from build123d import *

# Parameters (mm, degrees)
F0_W     = 10
F0_H     = 41.6184230894
F0_H_2   = 20
F1_DEPTH = 150
F2_W     = 6.3547044992
F2_H     = 150
F2_W_2   = 6.8435370922
F2_H_2   = 86.8458472192
F3_DEPTH = 25


with BuildPart() as f1:
    # F0 (on Top) → F1 (new body)
    with BuildSketch(Plane.XY):
        with Locations((-14.8092108965, -1.3289477304)):
            Rectangle(F0_W, F0_H)
        with Locations((-14.8092108965, -32.1381592751)):
            Rectangle(F0_W, F0_H_2)
    extrude(amount=F1_DEPTH)

    # F2 (on face) → F3 (join)
    with BuildSketch(Plane.YZ.offset(-9.8092108965)):
        with Locations((10.3059485555, 75)):
            Rectangle(F2_W, F2_H)
        with Locations((-32.4661172926, 106.5770763904)):
            Rectangle(F2_W_2, F2_H_2)
    extrude(amount=F3_DEPTH)


solid = f1.part
Read the model definition and answer for the solid it produces. Units are mm, in the model's axes. A direction names the side the tool comes from. Coordinates: 2 decimals unless noted, no trailing zeros. Order: outer loops, then holes, each group sorted by start corner. A loop starts at its lowest first (then second) coordinate and runs counter-clockwise, first axis right, second up. Notation, with made-up numbers: M 44,10.25 L 92,10.25 A24 ccw 92,48.25 Z; hole C 51.5,18 d11. An arc over 180 degrees is marked long. Put each result on its own line as item: value. Start each with the question number.
Item 1: The mould has two halves that part along Y. Classify faces 1 (the face through (3, -29.044, 106)), 2 (the face through (-19.809, -11, 74)), 3 (the face through (-15, 19.48, 74)): +Y half, -Y half, draft (parallel to the pull), parting line (faces both ways), or undercut.
Item 2: Section B-B, the plane z = 22 is taken. Determine the outline of the cut face in (x, y).
Item 3: Section C-C, the plane z = 119.5 is taken. Determine the outline of the cut face in (x, y).
Item 4: Given pin 1 Ø4 at (y, z) = (-6, 72.5) entering from +X; pin 2 Ø5 at (x, z) = (0, 92) entering from +Y; pin 3 Ø5 at (x, z) = (-6, 79.5) entering from -Y, each flat-ended and moving along its own axis, determine where each tip first touches the part or whether it passes through.
Item 5: Consider probe 1 along Y at (x, z) = (-6, 127.5); probe 2 along X at (y, z) = (-14, 48); probe 3 along Y at (x, z) = (-6, 37.5). Determine where each line is inside the solid, lowest interval first. Write a range as [from, to].
Item 6: For faces 4 (the face through (3, 7.129, 74)), 5 (the face through (3, 13.483, 74)), 6 (the face through (-10, -11, 150)), 7 (the face through (3, -35.888, 106)), 8 (the face through (3, -33, 63.154)), determine the directions among +Z, -Z, +X, -X, +Y, -Y from which every point of the face is accessible in a straight line to the end or side of a thin tool.
Item 7: Section D-D, the plane y = -25.5 is taken. Determine the outline of the cut face in (x, z), plus the area to 3 significant figures.
Item 8: Section A-A, the plane x = -3.5 is taken. Determine the outline of the cut face in (y, z).
Computed:
1. face 1: undercut
1. face 2: draft
1. face 3: +Y half
2. outline: M -19.81,-42.14 L -9.81,-42.14 L -9.81,7.13 L 15.19,7.13 L 15.19,13.48 L -9.81,13.48 L -9.81,19.48 L -19.81,19.48 Z
3. outline: M -19.81,-42.14 L -9.81,-42.14 L -9.81,-35.89 L 15.19,-35.89 L 15.19,-29.04 L -9.81,-29.04 L -9.81,7.13 L 15.19,7.13 L 15.19,13.48 L -9.81,13.48 L -9.81,19.48 L -19.81,19.48 Z
4. pin 1: stops at x = -9.81
4. pin 2: stops at y = 13.48
4. pin 3: stops at y = -35.89
5. probe 1: y = [-35.89, -29.04], [7.13, 13.48]
5. probe 2: x = [-19.81, -9.81]
5. probe 3: y = [7.13, 13.48]
6. face 4: +Z, -Z, +X
6. face 5: +Z, -Z, +X, +Y
6. face 6: +Z, +X, -X, +Y, -Y
6. face 7: +Z, -Z, +X, -Y
6. face 8: -Z, +X, -Y
7. outline: M -19.81,0 L -9.81,0 L -9.81,150 L -19.81,150 Z
7. area: 1,500 mm2
8. outline: M -35.89,63.15 L -29.04,63.15 L -29.04,150 L -35.89,150 Z; M 7.13,0 L 13.48,0 L 13.48,150 L 7.13,150 Z
